Autodesk Inventor part; units mm, degrees
ref_plane "WorkPlane1" through (0, 0, 0) normal (0, 0, 1) x (1, 0, 0)
ref_plane "MSC_PF1" through (0, 0, 0) normal (1, 0, 0) x (0, 1, 0)
ref_plane "MSC_PT1" through (0, 0, 0) normal (0, 0, -1) x (-1, 0, 0)
ref_plane "WorkPlane1" through (0, 0, 0) normal (0, 0, 1) x (1, 0, 0)
sketch "Sketch1" plane through (0, 0, 0) normal (0, 0, 1) x (1, 0, 0)
  point P0 (0, 0)
sketch "Sketch2" plane through (0, 0, 0) normal (0, 0, 1) x (1, 0, 0)
  line L0 (-4, 2.3095) -> (-4, -2.3095)
  line L1 (0, 4.6187) -> (-4, 2.3095)
  line L2 (4, 2.3095) -> (0, 4.6187)
  line L3 (4, -2.3095) -> (4, 2.3095)
  line L4 (0, -4.6187) -> (4, -2.3095)
  line L5 (-4, -2.3095) -> (0, -4.6187)
  circle A0 centre (0, 0) radius 4 construction
  dimension "d1" = 8
  dimension "d29" = 0
  dimension "d30" = 0
extrude "Extrusion1" add sketch "Sketch2" along normal blind 3.5
sketch "Sketch3" plane through (0, 0, 0) normal (1, 0, 0) x (0, 1, 0)
  line L0 (4, 3.5) -> (4.7187, 3.5)
  line L1 (4.7187, 3.085) -> (4, 3.5)
  line L2 (4.7187, 3.5) -> (4.7187, 3.085)
  line L3 (0, -0.7) -> (0, 4.2)
  line L4 (4.6187, 0) -> (4.6187, 3.5)
  dimension "d25" = 0.1
  dimension "d26" = 0
  dimension "d27" = 60
  dimension "d28" = 4
revolve "Revolution1" cut sketch "Sketch3" angle 360 about axis through (0, 0, -10) along (0, 0, 1)
sketch "Sketch4" plane through (0, 0, 0) normal (1, 0, 0) x (0, 1, 0)
  line L0 (0, -40) -> (0, 0)
  line L1 (-2.5, -40) -> (0, -40)
  line L2 (-2.5, 0) -> (-2.5, -40)
  line L3 (0, 0) -> (-2.5, 0)
  line L4 (0, -40) -> (0, 0)
  line L5 (-3, 0) -> (0.5, 0)
  line L6 (0, -48) -> (0, 8)
  dimension "d18" = 2.5
  dimension "d20" = 40
  dimension "d33" = 0
  dimension "d34" = 0
revolve "Revolution2" add sketch "Sketch4" angle 360 about axis through (0, 0, -40) along (0, 0, -1)
chamfer "Chamfer1" distance 0.4 angle 45 1 edges at (0, 2.5, -40)
fillet "Fillet1" radius 0.2 1 edges at (0, 2.5, 0)
thread "Thread1"
ref_plane "MSC_PF1" through (0, 0, 0) normal (1, 0, 0) x (0, 1, 0)
ref_plane "MSC_PT1" through (0, 0, 0) normal (0, 0, -1) x (-1, 0, 0)
equation "\"d22\" = 0.5 * PTC"
equation "\"d23\" = 0.5 * PTC"
equation "\"d24\" = r"
equation "\"d1\" = ParS"
equation "\"d6\" = ParK"
equation "\"b\" = NLG - 2 * PTC"
equation "\"d28\" = 0.5 * ParS"
equation "\"d18\" = 0.5 * NND"
equation "\"d20\" = NLG"
equation "\"NND\" = 5"
equation "\"NLG\" = 40"
equation "\"PTC\" = 0.8"
equation "\"ParK\" = 3.5"
equation "\"ParS\" = 8"
equation "\"msp_es\" = 0.577367 * ParS"
equation "\"r\" = 0.2"
equation "\"THREADDIA\" = NND"
properties part number "ISO 4018 - M5 x 40" material "Steel"
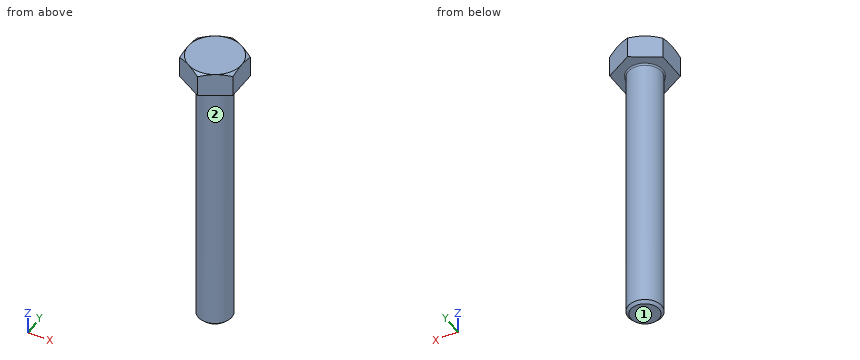
The listing builds one solid part. Answer for the finished solid, in the listing's coordinates (mm). Face numbers are marked on the shaded views. A direction names the side the tool comes from. Give positions to 0.01 mm unless a question says otherwise; leave off trailing zeros. Order: outer loops, then holes, each group sorted by start corner. A loop starts at its lowest first (then second) coordinate and runs counter-clockwise, first axis right, second up. Notation, with made-up numbers: (-17, -39.5) -> (22, -39.5) arc R24 cw to (22, -14.5) -> close; hole circle Ø6 at (35.5, 70). An arc over 180 degrees is marked (long way). Answer as a JSON object with one key per item and string values. Group by question number.
Item 1: A tool of negligible diameter and unlimited length cuts with its end or side. For the marked faces 1 and 2, from which of +Z, -Z, +X, -X, +Y, -Y can it reach the whole face along a straight path? Write none if from no direction.
Item 2: The part is cut by section A-A on z = -22.5. Write down the section's boundary in (x, y), and give its area (3 significant figures).
Item 3: Consider L1, parallel to Z at x = 1.75, y = -3; L2, parallel to Y at x = 1.5, z = -8; L3, parallel to Y at x = 0.5, z = -34.5. Determine where each line is inside the solid, lowest interval first. Write a range as from..to.
Item 4: A flat-ended cylindrical pin translates along its axis: pin 1 (3 mm diameter, centred on y = 3.5, z = -24, fed in from +X). Find the tip coordinate at first contact, or state that the pin passes through.
Result set:
{
 "1": {"face 1": "-Z, +X, -X, +Y, -Y", "face 2": "-Z"},
 "2": {"outline": "circle Ø5 at (0, 0)", "area": "19.6 mm²"},
 "3": {"L1": "0..3.5", "L2": "-2..2", "L3": "-2.45..2.45"},
 "4": {"pin 1": "x = 1.5"}
}
